Can you work these out from the model? Positions are in its coordinate system, mm. Give positions to 0.01 mm unless a question says otherwise; leave off trailing zeros. Order: outer loops, then holes, each group sorted by start corner. A loop starts at its lowest first (then second) coordinate and runs counter-clockwise, first axis right, second up. Notation, with made-up numbers: (22, -19.5) -> (29, -19.5) arc R28 ccw to (29, -0.5) -> close; hole circle Ø1 at (50.5, 58). An arc over 180 degrees is marked (long way). Answer as a JSON object with one key per item and string values.
```python
from build123d import *

# Parameters (mm, degrees)
F0_W     = 12.7
F0_H     = 6.35
F1_DEPTH = 3
F3_R     = 3.17499
F2_R     = 2.159
F4_DEPTH = 25.4


# Not quite as in the source:
# - a fillet or chamfer is up to 0.001 mm smaller than in the source, because OpenCascade refuses the exact size


with BuildPart() as f1:
    # F0 (on Top) → F1 (new body)
    with BuildSketch(Plane.XY):
        with Locations((6.35, 3.175)):
            Rectangle(F0_W, F0_H)
    extrude(amount=F1_DEPTH)

    # F3 (radius 3.175 in the source; OpenCascade refuses exactly that, so slightly less here)
    f3_edges = [f1.edges().sort_by_distance(p)[0] for p in [
        (12.7, 6.35, 1.5),
        (12.7, 0, 1.5),
    ]]
    fillet(f3_edges, radius=F3_R)

    # F2 (on face) → F4 (cut)
    with BuildSketch(Plane.XY.offset(3)):
        with Locations((8.9535, 3.175)):
            Circle(F2_R)
    extrude(amount=-F4_DEPTH, mode=Mode.SUBTRACT)


solid = f1.part
```
1. If we section it at C-C on y = 4.5: Please give me the cut outline in (x, z), then the cut area to 3 significant figures.
Worked answers:
{"outline": "(0, 0) -> (7.25, 0) -> (7.25, 3) -> (0, 3) -> close; (10.66, 0) -> (12.41, 0) -> (12.41, 3) -> (10.66, 3) -> close", "area": "27.0 mm²"}
2. Please list where these lines run through material, in increasing order: L1, parallel to X at y = 3.25, z = 1.55; L2, parallel to X at y = 4.5, z = 1.65; L3, parallel to Y at x = 7.75, z = 0.5.
Worked answers:
{"L1": "0 to 6.8, 11.11 to 12.7", "L2": "0 to 7.25, 10.66 to 12.41", "L3": "0 to 1.38, 4.97 to 6.35"}
3. If we mould it in two halves opening along X, with no side actions, what happens to faces 1 (the face through (7.24, 1.86, 1.52)), 2 (the face through (5, 0, 1)), 3 (the face through (0, 3, 1))? For each: +X half, -X half, draft (parallel to the pull), parting line (faces both ways), or undercut.
Worked answers:
{"face 1": "undercut", "face 2": "draft", "face 3": "-X half"}
4. If we section it at A-A on y = 2.25: Please give me the cut outline in (x, z), then the cut area to 3 significant figures.
Worked answers:
{"outline": "(0, 0) -> (7, 0) -> (7, 3) -> (0, 3) -> close; (10.9, 0) -> (12.56, 0) -> (12.56, 3) -> (10.9, 3) -> close", "area": "26.0 mm²"}
